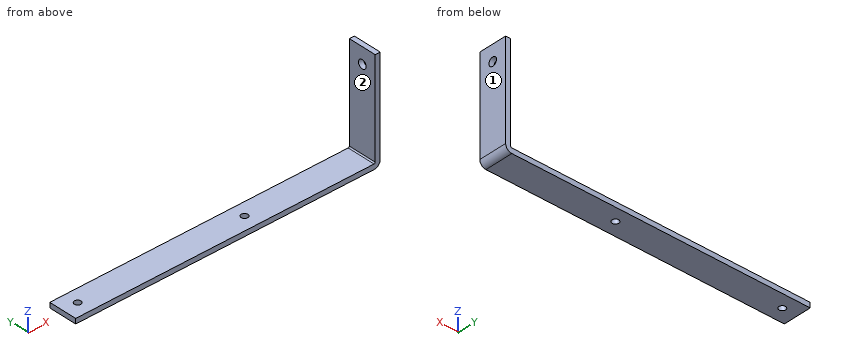
from build123d import *

# Parameters (mm, degrees)
SKETCH7_W                    = 190
SKETCH7_H                    = 18
BASE_FLANGE2_DEPTH           = 3.175
EDGE_FLANGE1_STRIP_W         = 14.1732
EDGE_FLANGE1_STRIP_H         = 3.175
EDGE_FLANGE1_STRIP_CUT_DEPTH = 18
EDGE_FLANGE1_DEPTH           = 18
M5X0_8_TAPPED_HOLE2_D        = 4.2
HOLE1_START                  = 190
HOLE1_OUTLINE_R              = 2.65
HOLE1_DEPTH                  = 3.175


# Read off the part's stored shape, not the designer's step: Hole1
# Sheet-metal steps are written as plain solids
with BuildPart() as part:
    # Sketch7 → Base-Flange2 (new body)
    with BuildSketch(Plane.XY):
        with Locations((95, 9)):
            Rectangle(SKETCH7_W, SKETCH7_H)
    extrude(amount=-BASE_FLANGE2_DEPTH)

    # Edge-Flange1 strip (across the edge) → Edge-Flange1 strip cut (cut)
    with BuildSketch(Plane(origin=(190, 0, 0), x_dir=(-1, 0, 0), z_dir=(0, 1, 0))):
        with Locations((-6.35, -1.5875)):
            Rectangle(EDGE_FLANGE1_STRIP_W, EDGE_FLANGE1_STRIP_H)
    extrude(amount=EDGE_FLANGE1_STRIP_CUT_DEPTH, mode=Mode.SUBTRACT)

    # Edge-Flange1 section (across the edge) → Edge-Flange1 (add)
    with BuildSketch(Plane(origin=(190, 0, 0), x_dir=(-1, 0, 0), z_dir=(0, 1, 0))):
        with BuildLine():
            Line((-3.175, 0.7366), (-3.175, 61.825))
            Line((-3.175, 61.825), (0, 61.825))
            Line((0, 61.825), (0, 0.7366))
            ThreePointArc((0, 0.7366), (0.215745145, 0.215745145), (0.7366, 0))
            Line((0.7366, 0), (0.7366, -3.175))
            ThreePointArc((0.7366, -3.175), (-2.029318885, -2.029318885), (-3.175, 0.7366))
        make_face()
    extrude(amount=EDGE_FLANGE1_DEPTH)

    # M5x0.8 Tapped Hole2 (through all)
    with Locations(Plane.XY):
        with Locations((9.5, 9), (115.5, 9.202035326)):
            Hole(M5X0_8_TAPPED_HOLE2_D / 2)

    # Hole1 outline → Hole1 (cut)
    with BuildSketch(Plane.YZ.offset(HOLE1_START)):
        with Locations((9, 51.825)):
            Circle(HOLE1_OUTLINE_R)
    extrude(amount=HOLE1_DEPTH, mode=Mode.SUBTRACT)


solid = part.part
Could you check a few things on this model? Use its own coordinates, in mm. Face numbers are marked on the shaded views. A direction names the side the tool comes from. Give positions to 0.01 mm unless a question says otherwise; leave off trailing zeros. Order: outer loops, then holes, each group sorted by start corner. A loop starts at its lowest first (then second) coordinate and runs counter-clockwise, first axis right, second up. Notation, with made-up numbers: (-36.5, -38.75) - (-25.5, -38.75) arc R11 ccw to (-25.5, -21.75) - close; hole circle Ø10 at (85.5, -31). An arc over 180 degrees is marked (long way). One line per item, written item: value. Start each with the question number.
1. Imagine slicing it at C-C on x = 97. List the corners of the cut face in (y, z) for me (3 decimals), plus the area to 4 significant figures.
2. Imagine slicing it at B-B on z = 7. List the corners of the cut face in (x, y) for me (3 decimals), plus the area to 4 significant figures.
3. For the marked faces 1 and 2, which set-ups out of +Z, -Z, +X, -X, +Y, -Y let a thin tool reach every point of the face, with its end or its side?
4. If I drill on probe 1 along Y at (x, z) = (9.5, -1.6); probe 2 along Y at (x, z) = (115.5, -0.75); probe 3 along X at (y, z) = (16, 5) (3 decimals), over which ranges is the centre line in solid material (lowest first)?
5. Imagine slicing it at A-A on x = 9.5. List the corners of the cut face in (y, z) for me (3 decimals).
6. For P1, Ø1.5, axis at x = 163, y = 16, coming from the +Z side; P2, Ø5.5, axis at x = 9.5, y = 9, coming from the -Z side (3 decimals); P3, Ø10, axis at y = 7, z = 24.5, coming from the -X side; P4, Ø5, axis at y = 9, z = 51.825, coming from the -X side, each with a flat end and sliding along its axis, tell me the tip position at first contact or that it passes through.
Values:
1. outline: (0, -3.175) - (18, -3.175) - (18, 0) - (0, 0) - close
1. area: 57.15 mm²
2. outline: (190, 0) - (193.175, 0) - (193.175, 18) - (190, 18) - close
2. area: 57.15 mm²
3. face 1: +Z, -Z, +X, +Y, -Y
3. face 2: +Z, -X, +Y, -Y
4. probe 1: 0 to 6.9, 11.1 to 18
4. probe 2: 0 to 7.1, 11.3 to 18
4. probe 3: 190 to 193.175
5. outline: (0, -3.175) - (6.9, -3.175) - (6.9, 0) - (0, 0) - close; (11.1, -3.175) - (18, -3.175) - (18, 0) - (11.1, 0) - close
6. P1: z = 0
6. P2: z = -3.175
6. P3: x = 190
6. P4: through
